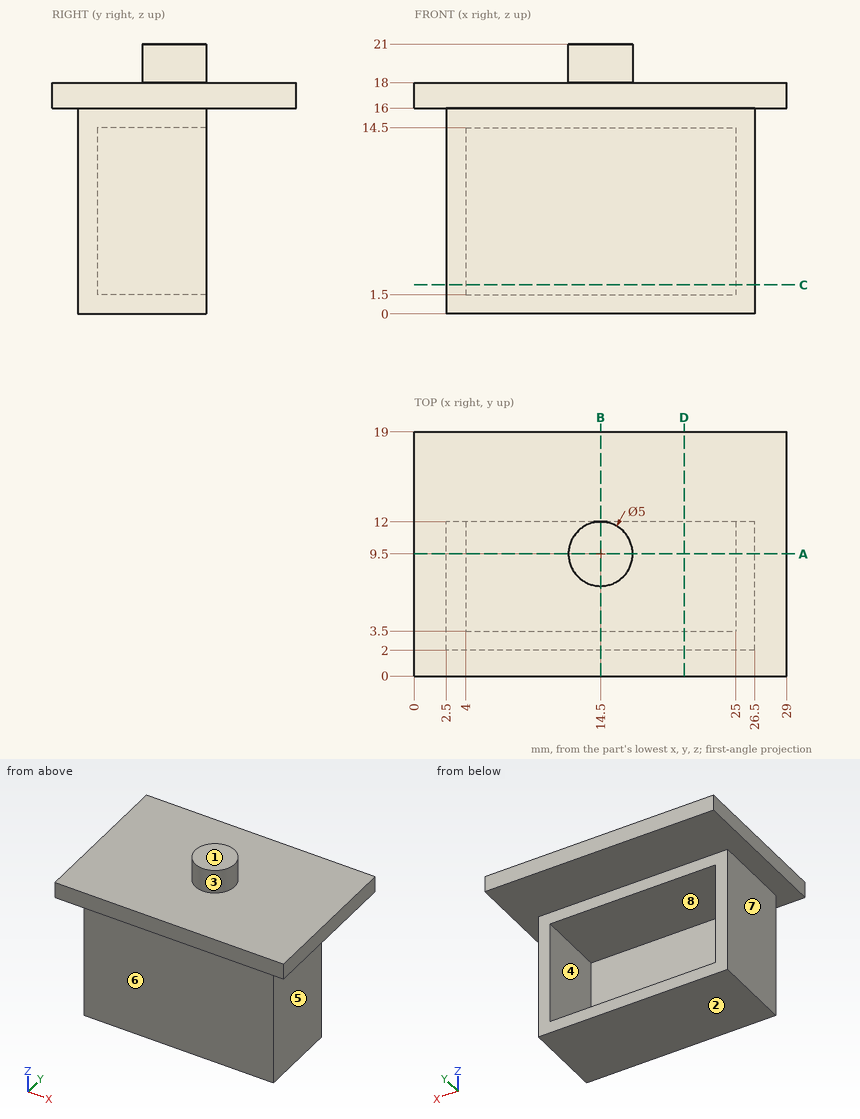
Study the drawing (mm; zero at the part's minimum x, y, z) and answer. A direction names the side the tool comes from. Give positions to 0.01 mm unless a question says otherwise; leave off trailing zeros. Loops run counter-clockwise (first coordinate to the right, second up) from the corner with the lowest first, then second, coordinate; pieces in that order, holes last. Notation, with made-up numbers: M 41,51 L 97,51 A24 cw 97,87 Z; hole C -5.75,59.5 d3. An arc over 180 degrees is marked long. One line per item, written item: value. Start each with the question number.
1. Determine the mould class of the marked faces 1, 2, 3 and 4 for opening direction Z: released by +Z, released by -Z, zero draft, split by the parting line, or undercut.
2. Find section A-A (y = 9.5). Give the vertices of the cut face in (x, z).
3. Find section D-D (x = 21). Give the vertices of the cut face in (y, z).
4. Each of these flat-tipped pins is pushed along its axis until it touches: P1, Ø4, axis at x = 17.5, z = 10.5, coming from the +Y side; P2, Ø11, axis at y = 6, z = 6, coming from the +X side; P3, Ø3, axis at y = 5, z = 8.5, coming from the -X side. Where does it stop, or does it pass through?
5. Find section B-B (x = 14.5). Give the vertices of the cut face in (y, z), and give its area (4 significant figures).
6. Find section C-C (z = 2.25). Give the vertices of the cut face in (x, y), and give its area (3 significant figures).
7. Which of the six approach directions +Z, -Z, +X, -X, +Y, -Y give full straight-line access (tool end or side, diameter ignored) to the marked faces 5, 6, 7 and 8?
8. Find the intervals of material crossed by probe 1 along X at (y, z) = (4.5, 4.5); probe 2 along Z at (x, y) = (4.5, 10.75); probe 3 along Z at (x, y) = (26, 15.5), in increasing order.
Reported:
1. face 1: released by +Z
1. face 2: released by -Z
1. face 3: zero draft
1. face 4: undercut
2. outline: M 0,16 L 2.5,16 L 2.5,0 L 26.5,0 L 26.5,16 L 29,16 L 29,18 L 17,18 L 17,21 L 12,21 L 12,18 L 0,18 Z; hole M 4,1.5 L 25,1.5 L 25,14.5 L 4,14.5 Z
3. outline: M 0,16 L 2,16 L 2,0 L 12,0 L 12,1.5 L 3.5,1.5 L 3.5,14.5 L 12,14.5 L 12,16 L 19,16 L 19,18 L 0,18 Z
4. P1: stops at y = 3.5
4. P2: stops at x = 26.5
4. P3: stops at x = 2.5
5. outline: M 0,16 L 2,16 L 2,0 L 12,0 L 12,1.5 L 3.5,1.5 L 3.5,14.5 L 12,14.5 L 12,16 L 19,16 L 19,18 L 12,18 L 12,21 L 7,21 L 7,18 L 0,18 Z
5. area: 102.5 mm²
6. outline: M 2.5,2 L 26.5,2 L 26.5,12 L 25,12 L 25,3.5 L 4,3.5 L 4,12 L 2.5,12 Z
6. area: 61.5 mm²
7. face 5: -Z, +X, +Y, -Y
7. face 6: -Z, +X, -X, -Y
7. face 7: -Z, -X, +Y, -Y
7. face 8: +Y
8. probe 1: x = 2.5 to 4, 25 to 26.5
8. probe 2: z = 0 to 1.5, 14.5 to 18
8. probe 3: z = 16 to 18
